Design review of the part built by this model. Coordinates are the model's own, in mm. Round coordinates to 2 decimals unless told otherwise and drop trailing zeros. Order: outer loops, then holes, each group sorted by start corner. A loop starts at its lowest first (then second) coordinate and runs counter-clockwise, first axis right, second up. Notation, with made-up numbers: M 32.25,68 L 48.25,68 A12 ccw 48.25,90 Z; hole C 12.5,62 d7. An arc over 180 degrees is marked long. Write each question's results on one line, items separated by ' | '. Start each with the question number.
Item 1: Wall thickness on line 1 (Z direction, x = -25.5, y = 1.8); line 2 (X direction, y = 1.9, z = 42.5): over which ranges is each line inside the solid? List them lowest first. Write a range as [from, to].
Item 2: Take a section at A-A, the plane z = 20. Write out the cut boundary in (x, y).
Item 3: Take a section at B-B, the plane x = -11.5. Count the separate pieces of the cut face and the enclosed holes in it, plus the area to 3 significant figures.
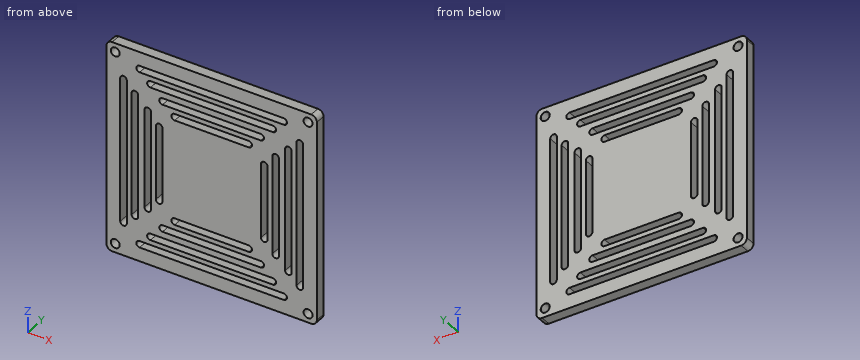
```python
from build123d import *

# Parameters (mm, degrees)
SKETCH1_W                       = 93.853
SKETCH1_H                       = 93.853
BOSS_EXTRUDE1_DEPTH             = 4.572
CUT_EXTRUDE1_DEPTH              = 67.521394968
F_4_0MM_DOWEL_HOLE1_D           = 4
F_4_0MM_DOWEL_HOLE1_CSINK_D     = 4.05
F_4_0MM_DOWEL_HOLE1_CSINK_ANGLE = 90
FILLET2_R                       = 2.54


with BuildPart() as part:
    # Sketch1 → Boss-Extrude1 (new body)
    with BuildSketch(Plane(origin=(0, 0, 0), x_dir=(1, 0, 0), z_dir=(0, 1, 0))):
        Rectangle(SKETCH1_W, SKETCH1_H)
    extrude(amount=BOSS_EXTRUDE1_DEPTH)

    # Sketch3 → Cut-Extrude1 (cut, through all)
    with BuildSketch(Plane(origin=(0, 4.572, 0), x_dir=(1, 0, 0), z_dir=(0, 1, 0))):
        with BuildLine():
            Line((-32.766, -27.305), (-32.766, 27.305))
            ThreePointArc((-32.766, 27.305), (-34.2265, 28.7655), (-35.687, 27.305))
            Line((-35.687, 27.305), (-35.687, -27.305))
            ThreePointArc((-35.687, -27.305), (-34.2265, -28.7655), (-32.766, -27.305))
        make_face()
        with BuildLine():
            Line((-27.051, -21.9075), (-27.051, 21.9075))
            ThreePointArc((-27.051, 21.9075), (-28.5115, 23.368), (-29.972, 21.9075))
            Line((-29.972, 21.9075), (-29.972, -21.9075))
            ThreePointArc((-29.972, -21.9075), (-28.5115, -23.368), (-27.051, -21.9075))
        make_face()
        with BuildLine():
            Line((-21.971, -16.51), (-21.971, 16.51))
            ThreePointArc((-21.971, 16.51), (-23.4315, 17.9705), (-24.892, 16.51))
            Line((-24.892, 16.51), (-24.892, -16.51))
            ThreePointArc((-24.892, -16.51), (-23.4315, -17.9705), (-21.971, -16.51))
        make_face()
        with BuildLine():
            Line((-16.51, 21.971), (16.51, 21.971))
            ThreePointArc((16.51, 21.971), (17.9705, 23.4315), (16.51, 24.892))
            Line((16.51, 24.892), (-16.51, 24.892))
            ThreePointArc((-16.51, 24.892), (-17.9705, 23.4315), (-16.51, 21.971))
        make_face()
        with BuildLine():
            Line((-21.9075, 27.051), (21.9075, 27.051))
            ThreePointArc((21.9075, 27.051), (23.368, 28.5115), (21.9075, 29.972))
            Line((21.9075, 29.972), (-21.9075, 29.972))
            ThreePointArc((-21.9075, 29.972), (-23.368, 28.5115), (-21.9075, 27.051))
        make_face()
        with BuildLine():
            Line((-27.305, 32.766), (27.305, 32.766))
            ThreePointArc((27.305, 32.766), (28.7655, 34.2265), (27.305, 35.687))
            Line((27.305, 35.687), (-27.305, 35.687))
            ThreePointArc((-27.305, 35.687), (-28.7655, 34.2265), (-27.305, 32.766))
        make_face()
        with BuildLine():
            Line((-32.131, 37.846), (32.131, 37.846))
            ThreePointArc((32.131, 37.846), (33.5915, 39.3065), (32.131, 40.767))
            Line((32.131, 40.767), (-32.131, 40.767))
            ThreePointArc((-32.131, 40.767), (-33.5915, 39.3065), (-32.131, 37.846))
        make_face()
        with BuildLine():
            Line((21.971, 16.51), (21.971, -16.51))
            ThreePointArc((21.971, -16.51), (23.4315, -17.9705), (24.892, -16.51))
            Line((24.892, -16.51), (24.892, 16.51))
            ThreePointArc((24.892, 16.51), (23.4315, 17.9705), (21.971, 16.51))
        make_face()
        with BuildLine():
            Line((27.051, 21.9075), (27.051, -21.9075))
            ThreePointArc((27.051, -21.9075), (28.5115, -23.368), (29.972, -21.9075))
            Line((29.972, -21.9075), (29.972, 21.9075))
            ThreePointArc((29.972, 21.9075), (28.5115, 23.368), (27.051, 21.9075))
        make_face()
        with BuildLine():
            Line((32.766, 27.305), (32.766, -27.305))
            ThreePointArc((32.766, -27.305), (34.2265, -28.7655), (35.687, -27.305))
            Line((35.687, -27.305), (35.687, 27.305))
            ThreePointArc((35.687, 27.305), (34.2265, 28.7655), (32.766, 27.305))
        make_face()
        with BuildLine():
            Line((37.846, 32.131), (37.846, -32.131))
            ThreePointArc((37.846, -32.131), (39.3065, -33.5915), (40.767, -32.131))
            Line((40.767, -32.131), (40.767, 32.131))
            ThreePointArc((40.767, 32.131), (39.3065, 33.5915), (37.846, 32.131))
        make_face()
        with BuildLine():
            Line((16.51, -21.971), (-16.51, -21.971))
            ThreePointArc((-16.51, -21.971), (-17.9705, -23.4315), (-16.51, -24.892))
            Line((-16.51, -24.892), (16.51, -24.892))
            ThreePointArc((16.51, -24.892), (17.9705, -23.4315), (16.51, -21.971))
        make_face()
        with BuildLine():
            Line((21.9075, -27.051), (-21.9075, -27.051))
            ThreePointArc((-21.9075, -27.051), (-23.368, -28.5115), (-21.9075, -29.972))
            Line((-21.9075, -29.972), (21.9075, -29.972))
            ThreePointArc((21.9075, -29.972), (23.368, -28.5115), (21.9075, -27.051))
        make_face()
        with BuildLine():
            Line((27.305, -32.766), (-27.305, -32.766))
            ThreePointArc((-27.305, -32.766), (-28.7655, -34.2265), (-27.305, -35.687))
            Line((-27.305, -35.687), (27.305, -35.687))
            ThreePointArc((27.305, -35.687), (28.7655, -34.2265), (27.305, -32.766))
        make_face()
        with BuildLine():
            Line((32.131, -37.846), (-32.131, -37.846))
            ThreePointArc((-32.131, -37.846), (-33.5915, -39.3065), (-32.131, -40.767))
            Line((-32.131, -40.767), (32.131, -40.767))
            ThreePointArc((32.131, -40.767), (33.5915, -39.3065), (32.131, -37.846))
        make_face()
        with BuildLine():
            Line((-40.767, -32.131), (-40.767, 32.131))
            ThreePointArc((-40.767, 32.131), (-39.3065, 33.5915), (-37.846, 32.131))
            Line((-37.846, 32.131), (-37.846, -32.131))
            ThreePointArc((-37.846, -32.131), (-39.3065, -33.5915), (-40.767, -32.131))
        make_face()
    extrude(amount=-CUT_EXTRUDE1_DEPTH, mode=Mode.SUBTRACT)

    # Ø4.0mm Dowel Hole1 (through all)
    with Locations(Plane(origin=(-42.9895, 4.572, 42.9895), x_dir=(0, 0, 1), z_dir=(0, 1, 0))):
        with Locations((0, 0), (-85.979, 0), (-85.979, 85.979), (0, 85.979)):
            CounterSinkHole(F_4_0MM_DOWEL_HOLE1_D / 2, F_4_0MM_DOWEL_HOLE1_CSINK_D / 2, counter_sink_angle=F_4_0MM_DOWEL_HOLE1_CSINK_ANGLE)

    # Fillet2
    fillet2_edges = [part.edges().sort_by_distance(p)[0] for p in [
        (-46.9265, 2.286, 46.9265),
        (46.9265, 2.286, 46.9265),
        (46.9265, 2.286, -46.9265),
        (-46.9265, 2.286, -46.9265),
    ]]
    fillet(fillet2_edges, radius=FILLET2_R)


solid = part.part
```
Results list:
1) line 1: [-46.93, -40.77], [-37.85, -35.69], [-32.77, 32.77], [35.69, 37.85], [40.77, 46.93] | line 2: [-46.93, -44.93], [-41.05, 41.05], [44.93, 46.93]
2) outline: M -46.93,0 L -40.77,0 L -40.77,4.57 L -46.93,4.57 Z; M -37.85,0 L -35.69,0 L -35.69,4.57 L -37.85,4.57 Z; M -32.77,0 L -29.97,0 L -29.97,4.57 L -32.77,4.57 Z; M -27.05,0 L 27.05,0 L 27.05,4.57 L -27.05,4.57 Z; M 29.97,0 L 32.77,0 L 32.77,4.57 L 29.97,4.57 Z; M 35.69,0 L 37.85,0 L 37.85,4.57 L 35.69,4.57 Z; M 40.77,0 L 46.93,0 L 46.93,4.57 L 40.77,4.57 Z
3) separate pieces: 9 | enclosed holes: 0 | area: 322 mm²
